The listing builds one solid part. Answer for the finished solid, in the listing's coordinates (mm). A direction names the side the tool comes from. Coordinates: 2 decimals unless noted, no trailing zeros. Order: outer loops, then holes, each group sorted by start corner. A loop starts at its lowest first (then second) coordinate and runs counter-clockwise, first axis right, second up. Notation, with made-up numbers: (66.5, 16.25) - (120.5, 16.25) arc R22 ccw to (120.5, 53.25) - close; hole circle Ø1 at (11.25, 52). An arc over 180 degrees is marked (long way). Use one line per item in the form item = value. Start each with the question number.
Item 1: Section A-A, the plane x = 11.3 is taken. Write down the section's boundary in (y, z).
Item 2: A tool of negligible diameter and unlimited length cuts with its end or side. For faces 1 (the flat face through (46.77, 2.46, -34.48)), 2 (the flat face through (52, 2, 0)), from which of +Z, -Z, +X, -X, +Y, -Y can it reach the whole face along a straight path? Write none if from no direction.
Item 3: Section B-B, the plane y = 2.45 is taken. Count the separate pieces of the cut face and the enclosed holes in it, and give its area (3 significant figures).
Item 4: This flat-tipped pin is pushed along its axis until it touches: pin 1 Ø2.5 at (x, z) = (11.3, -2.6) entering from +Y. Where does it stop, or does it pass through?
Item 5: Consider line 1 along X through (y, z) = (3.65, -2.6); line 2 along X through (y, z) = (3.85, -63.1); line 3 along Z through (x, y) = (86.5, 2.1). Determine where each line is inside the solid, lowest interval first. Write a range as [from, to].
from build123d import *

# Parameters (mm, degrees)
CROQUIS1_R              = 1.7
SALIENTE_EXTRUIR1_DEPTH = 5


with BuildPart() as part:
    # Croquis1 → Saliente-Extruir1 (new body)
    with BuildSketch(Plane(origin=(0, 0, 0), x_dir=(1, 0, 0), z_dir=(0, 1, 0))):
        Polygon((0, 53.1), (0, 63.1), (10, 73.1), (92, 73.1), (102, 63.1), (102, 53.1), (102, 0), (0, 0), align=None)
        with Locations((7.35, 50.4)):
            Circle(CROQUIS1_R, mode=Mode.SUBTRACT)
        with Locations((11.3, 2.6)):
            Circle(CROQUIS1_R, mode=Mode.SUBTRACT)
        with Locations((86.5, 50.5)):
            Circle(CROQUIS1_R, mode=Mode.SUBTRACT)
        with Locations((86.5, 2.6)):
            Circle(CROQUIS1_R, mode=Mode.SUBTRACT)
        with Locations((25.5, 63.1)):
            Circle(CROQUIS1_R, mode=Mode.SUBTRACT)
        with Locations((76.5, 63.1)):
            Circle(CROQUIS1_R, mode=Mode.SUBTRACT)
        with BuildLine():
            Line((44.188139939, 41.934668839), (45.501537669, 43.270342848))
            Line((45.501537669, 43.270342848), (47.224863288, 42.26739732))
            ThreePointArc((47.224863288, 42.26739732), (47.575067996, 42.169782903), (47.928320792, 42.255715279))
            ThreePointArc((47.928320792, 42.255715279), (48.469957789, 42.515675688), (49.033343063, 42.724355067))
            ThreePointArc((49.033343063, 42.724355067), (49.340671144, 42.918574947), (49.513928995, 43.23818976))
            Line((49.513928995, 43.23818976), (49.990823409, 45.174248292))
            Line((49.990823409, 45.174248292), (51.864, 45.19))
            Line((51.864, 45.19), (52.373385647, 43.262235184))
            ThreePointArc((52.373385647, 43.262235184), (52.551993955, 42.945579245), (52.862544768, 42.756555163))
            ThreePointArc((52.862544768, 42.756555163), (53.429359729, 42.557379737), (53.975291881, 42.306564794))
            ThreePointArc((53.975291881, 42.306564794), (54.329939845, 42.226585218), (54.678453448, 42.330075218))
            Line((54.678453448, 42.330075218), (56.384668839, 43.361860061))
            Line((56.384668839, 43.361860061), (57.720342848, 42.048462331))
            Line((57.720342848, 42.048462331), (56.71739732, 40.325136712))
            ThreePointArc((56.71739732, 40.325136712), (56.619782903, 39.974932004), (56.705715279, 39.621679208))
            ThreePointArc((56.705715279, 39.621679208), (56.965675688, 39.080042211), (57.174355067, 38.516656937))
            ThreePointArc((57.174355067, 38.516656937), (57.368574947, 38.209328856), (57.68818976, 38.036071005))
            Line((57.68818976, 38.036071005), (59.624248292, 37.559176591))
            Line((59.624248292, 37.559176591), (59.64, 35.686))
            Line((59.64, 35.686), (57.712235184, 35.176614353))
            ThreePointArc((57.712235184, 35.176614353), (57.395579245, 34.998006045), (57.206555163, 34.687455232))
            ThreePointArc((57.206555163, 34.687455232), (57.007379737, 34.120640271), (56.756564794, 33.574708119))
            ThreePointArc((56.756564794, 33.574708119), (56.676585218, 33.220060155), (56.780075218, 32.871546552))
            Line((56.780075218, 32.871546552), (57.811860061, 31.165331161))
            Line((57.811860061, 31.165331161), (56.498462331, 29.829657152))
            Line((56.498462331, 29.829657152), (54.775136712, 30.83260268))
            ThreePointArc((54.775136712, 30.83260268), (54.424932004, 30.930217097), (54.071679208, 30.844284721))
            ThreePointArc((54.071679208, 30.844284721), (53.530042211, 30.584324312), (52.966656937, 30.375644933))
            ThreePointArc((52.966656937, 30.375644933), (52.724095072, 30.403806003), (52.486071005, 30.349273006))
            Line((52.486071005, 30.349273006), (52.009176591, 28.413214474))
            Line((52.009176591, 28.413214474), (50.136, 28.397462767))
            Line((50.136, 28.397462767), (49.626614353, 30.325227583))
            ThreePointArc((49.626614353, 30.325227583), (49.383630447, 30.377181799), (49.137455232, 30.343444837))
            ThreePointArc((49.137455232, 30.343444837), (48.570640271, 30.542620263), (48.024708119, 30.793435206))
            ThreePointArc((48.024708119, 30.793435206), (47.670060155, 30.873414782), (47.321546552, 30.769924782))
            Line((47.321546552, 30.769924782), (45.615331161, 29.738139939))
            Line((45.615331161, 29.738139939), (44.279657152, 31.051537669))
            Line((44.279657152, 31.051537669), (45.28260268, 32.774863288))
            ThreePointArc((45.28260268, 32.774863288), (45.380217097, 33.125067996), (45.294284721, 33.478320792))
            ThreePointArc((45.294284721, 33.478320792), (45.208247472, 33.643799276), (45.127008205, 33.811685303))
            ThreePointArc((45.127008205, 33.811685303), (45.125953752, 33.923547873), (45.209575503, 33.997856347))
            Line((45.209575503, 33.997856347), (48.384042323, 34.978554615))
            ThreePointArc((48.384042323, 34.978554615), (54.05159058, 36.528318352), (48.406635637, 38.158457784))
            Line((48.406635637, 38.158457784), (45.170602247, 39.00232588))
            ThreePointArc((45.170602247, 39.00232588), (45.082937198, 39.074508031), (45.08129489, 39.188054174))
            ThreePointArc((45.08129489, 39.188054174), (45.159930296, 39.35784363), (45.243435206, 39.525291881))
            ThreePointArc((45.243435206, 39.525291881), (45.323414782, 39.879939845), (45.219924782, 40.228453448))
            Line((45.219924782, 40.228453448), (44.188139939, 41.934668839))
        make_face(mode=Mode.SUBTRACT)
    extrude(amount=SALIENTE_EXTRUIR1_DEPTH)


solid = part.part
Response:
q1.outline = (0, -73.1) - (5, -73.1) - (5, -4.3) - (0, -4.3) - close; (0, -0.9) - (5, -0.9) - (5, 0) - (0, 0) - close
q2.face_1 = +Y, -Y
q2.face_2 = +Z, +X, -X, +Y, -Y
q3.separate_pieces = 1
q3.enclosed_holes = 7
q3.area = 7,180 mm2
q4.pin_1 = through
q5.line_1 = [0, 9.6], [13, 84.8], [88.2, 102]
q5.line_2 = [0, 23.8], [27.2, 74.8], [78.2, 102]
q5.line_3 = [-73.1, -52.2], [-48.8, -4.3], [-0.9, 0]
